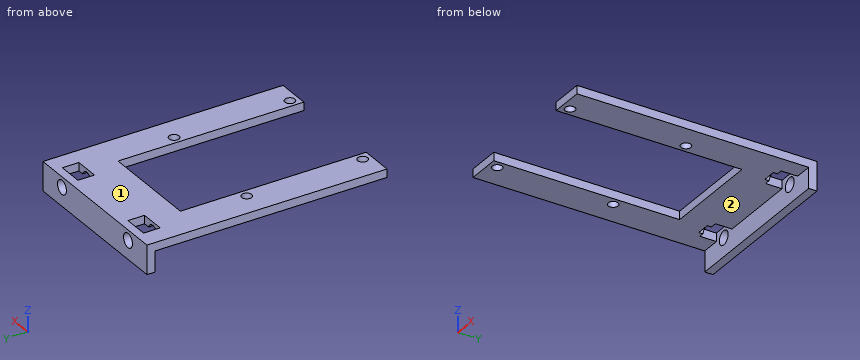
from build123d import *

# Parameters (mm, degrees)
SKETCH_W        = 40
SKETCH_H        = 58
PAD_DEPTH       = 2
SKETCH001_W     = 24
SKETCH001_H     = 50
POCKET_DEPTH    = 5
SKETCH002_W     = 40
SKETCH002_H     = 2
PAD001_DEPTH    = 5
SKETCH004_R     = 1.7
POCKET001_DEPTH = 7
SKETCH005_R     = 1.2
POCKET002_DEPTH = 5
SKETCH006_W     = 6
SKETCH006_H     = 4
POCKET003_DEPTH = 5
SKETCH007_R     = 1.2
POCKET004_DEPTH = 5


with BuildPart() as part:
    # Sketch → Pad (new body)
    with BuildSketch(Plane.XY):
        Rectangle(SKETCH_W, SKETCH_H)
    extrude(amount=PAD_DEPTH)

    # Sketch001 (on Face6 of Pad) → Pocket (cut)
    with BuildSketch(Plane.XY.offset(2)):
        with Locations((0, -9.102527)):
            Rectangle(SKETCH001_W, SKETCH001_H)
    extrude(amount=-POCKET_DEPTH, mode=Mode.SUBTRACT)

    # Sketch002 (on Face4 of Pocket) → Pad001 (join)
    with BuildSketch(Plane(origin=(0, 0, 0), x_dir=(1, 0, 0), z_dir=(0, 0, -1))):
        with Locations((0, -28)):
            Rectangle(SKETCH002_W, SKETCH002_H)
    extrude(amount=PAD001_DEPTH)

    # Sketch004 (on Face4 of Pad001) → Pocket001 (cut)
    with BuildSketch(Plane(origin=(0, 29, 0), x_dir=(-1, 0, 0), z_dir=(0, 1, 0))):
        with Locations((-12.71, -0.5)):
            Circle(SKETCH004_R)
        with Locations((12.71, -0.5)):
            Circle(SKETCH004_R)
    extrude(amount=-POCKET001_DEPTH, mode=Mode.SUBTRACT)

    # Sketch005 (on Face5 of Pocket001) → Pocket002 (cut)
    with BuildSketch(Plane.YZ.offset(20)):
        with Locations((-14, 25)):
            Circle(SKETCH005_R)
        with Locations((14, 25)):
            Circle(SKETCH005_R)
        with Locations((14, -3)):
            Circle(SKETCH005_R)
        with Locations((-14, -3)):
            Circle(SKETCH005_R)
    extrude(amount=-POCKET002_DEPTH, mode=Mode.SUBTRACT)

    # Sketch006 (on Face12 of Pocket002) → Pocket003 (cut)
    with BuildSketch(Plane(origin=(0, 0, 0), x_dir=(1, 0, 0), z_dir=(0, 0, -1))):
        with Locations((-12.517092, -25)):
            Rectangle(SKETCH006_W, SKETCH006_H)
        with Locations((12.746344, -25)):
            Rectangle(SKETCH006_W, SKETCH006_H)
    extrude(amount=-POCKET003_DEPTH, mode=Mode.SUBTRACT)

    # Sketch007 (on Face15 of Pocket003) → Pocket004 (cut)
    with BuildSketch(Plane(origin=(0, 0, 0), x_dir=(1, 0, 0), z_dir=(0, 0, -1))):
        with Locations((-14, 26.898312)):
            Circle(SKETCH007_R)
        with Locations((14, 26.898312)):
            Circle(SKETCH007_R)
        with Locations((14, -1.101688)):
            Circle(SKETCH007_R)
        with Locations((-14, -1.101688)):
            Circle(SKETCH007_R)
    extrude(amount=-POCKET004_DEPTH, mode=Mode.SUBTRACT)


solid = part.part
Model file for the job. Use its own axes, mm. Face numbers are marked on the shaded views. A direction names the side the tool comes from. Give positions to 0.01 mm unless a question says otherwise; leave off trailing zeros. Write each loop counter-clockwise with the first axis right and the second up, starting at its lowest first coordinate (ties: lowest second). Pieces come first, ordered by that corner, then holes. Notation, with made-up numbers: M -20,83.25 L -13,83.25 A27 ccw -13,117.25 Z; hole C -8.5,79.25 d4. An arc over 180 degrees is marked long. One line per item, written item: value. Start each with the question number.
Q1. Probe probe 1 along Y at (x, z) = (14, 1.3); probe 2 along Z at (x, y) = (-12.71, 27.6); probe 3 along Y at (x, z) = (-14, 0.55). List the from-to ranges inside material, lowest first. Write a range as [from, to].
Q2. Saw through at B-B, the plane x = -16.5. Write the cut outline in (y, z), plus the area to 3 significant figures.
Q3. Saw through at A-A, the plane y = 6. Write the cut outline in (x, z).
Q4. Saw through at C-C, the plane z = -3.75. Write the cut outline in (x, y), plus the area to 3 significant figures.
Q5. 3-axis set-ups, long thin cutter, end or side, ignore diameter. For the marked faces 1 and 2: which of +Z, -Z, +X, -X, +Y, -Y reach the whole face in a straight line?
Q6. Saw through at D-D, the plane x = 7.5. Write the cut outline in (y, z), plus the area to 3 significant figures.
Q7. Drop flat-ended pins along their axis: pin 1 Ø4 at (x, z) = (12.71, -0.5) entering from +Y; pin 2 Ø4 at (x, y) = (-15, -1) entering from -Z; pin 3 Ø0.6 at (x, z) = (13.5, 0.5) entering from +Y. Give the stop position or say it passes through.
Output values:
1. probe 1: y = [-29, -28.1], [-25.7, -0.1], [2.3, 23], [27, 29]
1. probe 2: z = [-5, -2.2], [1.2, 2]
1. probe 3: y = [-29, -28.1], [-25.7, -0.1], [2.3, 22]
2. outline: M -29,0 L 27,0 L 27,-5 L 29,-5 L 29,2 L -29,2 Z
2. area: 126 mm²
3. outline: M -20,0 L -12,0 L -12,2 L -20,2 Z; M 12,0 L 20,0 L 20,2 L 12,2 Z
4. outline: M -20,27 L 20,27 L 20,29 L -20,29 Z
4. area: 80.0 mm²
5. face 1: +Z, +X, -X, +Y, -Y
5. face 2: -Z, +X, -X, -Y
6. outline: M 15.9,0 L 27,0 L 27,-5 L 29,-5 L 29,2 L 15.9,2 Z
6. area: 36.2 mm²
7. pin 1: stops at y = 29
7. pin 2: stops at z = 0
7. pin 3: stops at y = 22
